Autodesk Inventor part; units mm, degrees
ref_plane "YZ Plane" through (0, 0, 0) normal (1, 0, 0) x (0, 1, 0)
ref_plane "XZ Plane" through (0, 0, 0) normal (0, 1, 0) x (-1, 0, 0)
ref_plane "XY Plane" through (0, 0, 0) normal (0, 0, 1) x (1, 0, 0)
sketch "Sketch1" plane through (0, 0, 0) normal (0, 1, 0) x (-1, 0, 0)
  line L0 (0, 0) -> (150, 0)
  line L1 (150, 0) -> (150, 100)
  line L2 (150, 100) -> (0, 100)
  line L3 (0, 100) -> (0, 0)
  dimension "d0" = 150
  dimension "d1" = 100
extrude "Extrusion1" add sketch "Sketch1" along normal blind 20
sketch "Sketch2" plane through (0, 20, 0) normal (0, 1, 0) x (1, 0, 0)
  point P0 (0, 0)
sketch "Sketch3" plane through (0, 20, 0) normal (0, 1, 0) x (1, 0, 0)
  point P0 (0, 0)
sketch "Sketch4" plane through (0, 20, 0) normal (0, 1, 0) x (1, 0, 0)
  line L0 (-88.5149, -68.8546) -> (-50.8129, -68.8546)
  line L1 (-50.8129, -68.8546) -> (-50.8129, -31.4381)
  line L2 (-50.8129, -31.4381) -> (-88.5149, -31.4381)
  line L3 (-88.5149, -31.4381) -> (-88.5149, -68.8546)
  point P0 (0, 0)
extrude "Extrusion2" add sketch "Sketch4" along normal blind 2
sketch "Sketch8" plane through (0, 22, 0) normal (0, 1, 0) x (1, 0, 0)
  point P0 (0, 0)
sketch "Sketch9" plane through (0, 22, 0) normal (0, 1, 0) x (1, 0, 0)
  line L0 (-50.8129, -68.8546) -> (-88.5149, -68.8546)
  line L1 (-88.5149, -31.4381) -> (-50.8129, -31.4381)
  line L2 (-82.8248, -68.8546) -> (-52.6097, -68.8546)
  line L3 (-52.6097, -68.8546) -> (-52.6097, -31.4381)
  line L4 (-52.6097, -31.4381) -> (-82.8248, -31.4381)
  line L5 (-82.8248, -31.4381) -> (-82.8248, -68.8546)
  point P0 (0, 0)
extrude "Extrusion5" add sketch "Sketch9" along normal blind 35
sketch "Sketch10" plane through (-82.8248, 22, 31.4381) normal (-1, 0, 0) x (0, 0, 1)
  line L0 (13.2287, 19.9432) -> (24.5588, 19.9432)
  line L1 (24.5588, 19.9432) -> (24.5588, 10.3562)
  line L2 (24.5588, 10.3562) -> (13.2287, 10.3562)
  line L3 (13.2287, 10.3562) -> (13.2287, 19.9432)
  point P0 (-31.4381, -22)
extrude "Extrusion6" add sketch "Sketch10" along normal blind 15
sketch "Sketch12" plane through (-82.8248, 32.3562, 44.6668) normal (0, 0, -1) x (-1, 0, 0)
  circle A0 centre (10.1482, 4.7576) radius 4.2682
  point P0 (-82.8248, -32.3562)
extrude "Extrusion7" add sketch "Sketch12" along normal blind 180
sketch "Sketch13" plane through (-97.8248, 22, 31.4381) normal (-1, 0, 0) x (0, 0, 1)
  point P0 (-31.4381, -22)
sketch "Sketch14" plane through (0, 0, 0) normal (0, 0, 1) x (1, 0, 0)
  point P0 (0, 0)
sketch "Sketch15" plane through (0, 0, 0) normal (0, 1, 0) x (-1, 0, 0)
  point P0 (0, 0)
sketch "Sketch16" plane through (0, 0, 0) normal (0, 1, 0) x (-1, 0, 0)
  point P0 (0, 0)
sketch "Sketch17" plane through (-92.973, 37.1137, -135.3332) normal (0, 0, -1) x (-1, 0, 0)
  circle A0 centre (0, 0) radius 4.2682
  point P0 (-92.973, -37.1137)
sketch "Sketch18" plane through (-92.973, 37.1137, -135.3332) normal (0, 0, -1) x (-1, 0, 0)
  point P0 (-92.973, -37.1137)
sketch "Sketch19" plane through (-92.973, 37.1137, -135.3332) normal (0, 0, -1) x (-1, 0, 0)
  point P0 (-92.973, -37.1137)
sketch "Sketch20" plane through (-92.973, 37.1137, -135.3332) normal (0, 0, -1) x (-1, 0, 0)
  line L0 (-2.448, 2.726) -> (2.3625, 2.726)
  line L1 (2.3625, 2.726) -> (2.3625, -2.6968)
  line L2 (2.3625, -2.6968) -> (-2.448, -2.6968)
  line L3 (-2.448, -2.6968) -> (-2.448, 2.726)
  point P0 (-92.973, -37.1137)
extrude "Extrusion8" add sketch "Sketch20" along normal blind 8
sketch "Sketch21" plane through (-95.3355, 34.417, -135.3332) normal (0, -1, 0) x (1, 0, 0)
  point P0 (95.3355, 135.3332)
sketch "Sketch22" plane through (-95.3355, 34.417, -135.3332) normal (0, -1, 0) x (1, 0, 0)
  point P0 (95.3355, 135.3332)
sketch "Sketch23" plane through (-95.3355, 34.417, -135.3332) normal (0, -1, 0) x (1, 0, 0)
  line L0 (0, -8) -> (4.8105, -8)
  line L1 (-1.9057, 0) -> (6.6307, 0)
  line L2 (0, -8) -> (4.9417, -8)
  line L3 (4.9417, -8) -> (4.9417, 0)
  line L4 (4.9417, 0) -> (0, 0)
  line L5 (0, 0) -> (0, -8)
  point P0 (95.3355, 135.3332)
extrude "Extrusion9" add sketch "Sketch23" along normal blind 70
sketch "Sketch27" plane through (0, 0, 100) normal (1, 0, 0) x (0, 0, -1)
  line L0 (0, 0) -> (100, 0)
  line L1 (100, 0) -> (50, 0)
  line L2 (100, 0) -> (0, 0)
  line L3 (75, 0) -> (50, 0)
  line L4 (0, 0) -> (50, 0)
  circle A0 centre (25, 0) radius 6
  circle A1 centre (50, 0) radius 6
  circle A2 centre (75, 0) radius 6
  dimension "d24" = 12
  dimension "d25" = 12
  dimension "d26" = 12
extrude "Extrusion10" cut sketch "Sketch27" along normal through all both and the other way through all
sketch "Sketch30" plane through (0, 57, 0) normal (0, 1, 0) x (1, 0, 0)
  line L0 (-150, -31) -> (0, -31)
  line L1 (-85.8103, -31) -> (-48.4742, -31)
  line L2 (-48.4742, -31) -> (-48.4742, -68.8679)
  line L3 (-48.4742, -68.8679) -> (-85.8103, -68.8679)
  line L4 (-85.8103, -68.8679) -> (-85.8103, -31)
  point P0 (0, 0)
extrude "Extrusion11" add sketch "Sketch30" along normal blind 2
sketch "Sketch31" plane through (0, 20, 0) normal (0, 1, 0) x (1, 0, 0)
  line L0 (0, -69) -> (-150, -69)
  line L1 (-150, -31) -> (0, -31)
  line L2 (-49.8943, -69) -> (-47.9179, -69)
  line L3 (-47.9179, -69) -> (-47.9179, -31)
  line L4 (-47.9179, -31) -> (-49.8943, -31)
  line L5 (-49.8943, -31) -> (-49.8943, -69)
  point P0 (0, 0)
extrude "Extrusion12" add sketch "Sketch31" along normal blind 40
sketch "Sketch32" plane through (0, 59, 0) normal (0, 1, 0) x (1, 0, 0)
  circle A0 centre (-83.7761, -33.1539) radius 1.2799
  circle A1 centre (-83.7761, -66.902) radius 1.3017
  point P0 (0, 0)
extrude "Extrusion13" cut sketch "Sketch32" against normal blind 40
sketch "Sketch33" plane through (-47.9179, 20, 69) normal (1, 0, 0) x (0, 0, -1)
  line L0 (0.1321, 37) -> (38, 37)
  circle A0 centre (34.1824, 37) radius 1.5602
  circle A1 centre (2.8109, 37) radius 1.6636
  point P0 (69, -20)
extrude "Extrusion14" cut sketch "Sketch33" against normal blind 40
properties part number "Vertical"
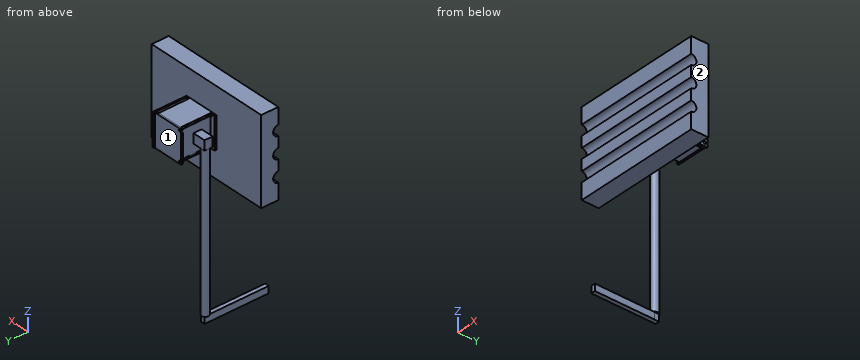
Source: CAD feature listing. Evaluate the final solid. Frame: model axes, mm. Face numbers are marked on the shaded views. A direction names the side the tool comes from. Round coordinates to 2 decimals unless told otherwise and drop trailing zeros. Write each loop counter-clockwise with the first axis right and the second up, starting at its lowest first coordinate (ties: lowest second). Pieces come first, ordered by that corner, then holes. Notation, with made-up numbers: (35.5, -2) - (53.5, -2) arc R26 cw to (53.5, 15) - close; hole circle Ø2 at (13.5, -36). An arc over 180 degrees is marked (long way). Use CSV: the item, a comma, the result in double quotes. Start each with the question number.
(1) Set-up query: the marked faces 1 and 2. Return all of +Z, -Z, +X, -X, +Y, -Y with unobstructed straight access to the full face (end or side cutting, diameter ignored); none if empty.
(2) Cut plane C-C, the plane y = 11. Return loops of the section in (x, z).
(3) Material intervals for probe 1 along Z at (x, y) = (-31, 3); probe 2 along Z at (x, y) = (-141, 7.5); probe 3 along Y at (x, z) = (-88.5, 83.5), sorted ascending. Write a range as [from, to].
(4) Cut plane B-B, the plane x = -76. Give the number of separate pieces and of enclosed holes in the cut face, and give its area (3 significant figures).
(5) First-contact query: pin 1 Ø3.5 at (x, z) = (-83.78, 66.9) entering from +Y; pin 2 Ø1 at (y, z) = (21.5, 52) entering from -X; pin 3 Ø0.8 at (x, z) = (-51.5, 48) entering from -Y. Flat tips, straight axial feed; report the tip coordinate or a pass-through.
(6) Cut plane A-A, the plane z = 50. Return loops of the section in (x, y), and give its area (3 significant figures).
(7) Cut plane D-D, the plane x = -26. Return loops of the section in (y, z).
Geometry says:
1,face 1,"+Z, -Z, -X, +Y"
1,face 2,"+Z, -Z, +X, +Y, -Y"
2,outline,"(-150, 0) - (0, 0) - (0, 100) - (-150, 100) - close; (-95.34, -143.33) - (-90.39, -143.33) - (-90.39, -135.33) - (-95.34, -135.33) - close"
3,probe 1,"[0, 19.8], [30.2, 44.8], [55.2, 69.8], [80.2, 100]"
3,probe 2,"[0, 100]"
3,probe 3,"[0, 20]"
4,separate pieces,"1"
4,enclosed holes,"2"
4,area,"3,270 mm²"
5,pin 1,"y = 59"
5,pin 2,"x = -88.51"
5,pin 3,"y = 5.5"
6,outline,"(-150, 6) - (0, 6) - (0, 20) - (-47.92, 20) - (-47.92, 60) - (-49.89, 60) - (-49.89, 59) - (-85.81, 59) - (-85.81, 57) - (-82.82, 57) - (-82.82, 41.94) - (-97.82, 41.94) - (-97.82, 32.36) - (-82.82, 32.36) - (-82.82, 22) - (-88.51, 22) - (-88.51, 20) - (-150, 20) - close; hole (-52.61, 22) - (-50.81, 22) - (-50.81, 20) - (-49.89, 20) - (-49.89, 57) - (-52.61, 57) - close"
6,area,"3,530 mm²"
7,outline,"(0, 0) - (20, 0) - (20, 100) - (0, 100) - (0, 81) arc R6 cw to (0, 69) - (0, 56) arc R6 cw to (0, 44) - (0, 31) arc R6 cw to (0, 19) - close"
